```python
from build123d import *

# Parameters (mm, degrees)
SKETCH1_W                = 20
SKETCH1_H                = 15
SWITCHCASE_DEPTH         = 15
SKETCH2_W                = 12.9
SKETCH2_H                = 5.9
SWITCHCAVITY_DEPTH       = 30.154759474
SWITCHM2HOLES_DEPTH      = 28.096171316
SWITCHM2HOLES_DEPTH_BACK = 28.096171316
SKETCH3_R                = 1.05
NUTINSERTS_DEPTH         = 30.154759474
NUTINSERTS_DEPTH_BACK    = 1.75
SKETCH4_W                = 10
SKETCH4_H                = 10
MOUNTTABS_DEPTH          = 2.5
M5SCREWHOLES_REACH       = 36.369
SKETCH6_R                = 2.75
WINGS_DEPTH              = 15
WIRECHANNEL_DEPTH        = 43.884758365
WIRECHANNEL_DEPTH_BACK   = 43.884758365
SKETCH8_W                = 3
SKETCH8_H                = 3
BUMPERCHANNEL_DEPTH      = 46.552167896
BUMPERCHANNEL_DEPTH_BACK = 10.45


with BuildPart() as part:
    # Sketch1 → SwitchCase (new body)
    with BuildSketch(Plane.XY):
        with Locations((10, 7.5)):
            Rectangle(SKETCH1_W, SKETCH1_H)
    extrude(amount=SWITCHCASE_DEPTH)

    # Sketch2 → SwitchCavity (cut, through all)
    with BuildSketch(Plane(origin=(0, 15, 0), x_dir=(1, 0, 0), z_dir=(0, 1, 0))):
        with Locations((10, -7.5)):
            Rectangle(SKETCH2_W, SKETCH2_H)
    extrude(amount=-SWITCHCAVITY_DEPTH, mode=Mode.SUBTRACT)

    # Sketch3 → SwitchM2Holes (cut, two sides: drawn at the far end of the back side and taken through both)
    with BuildSketch(Plane.XY.offset(4.55).offset(-SWITCHM2HOLES_DEPTH_BACK)):
        with Locations((6.7, 8.9)):
            Circle(SKETCH3_R)
        with Locations((13.3, 8.9)):
            Circle(SKETCH3_R)
    extrude(amount=SWITCHM2HOLES_DEPTH + SWITCHM2HOLES_DEPTH_BACK, mode=Mode.SUBTRACT)

    # Sketch5 → NutInserts (cut, two sides: drawn at the far end of the back side and taken through both)
    with BuildSketch(Plane.XY.offset(15).offset(-NUTINSERTS_DEPTH_BACK)):
        Polygon((9.009401077, 8.9), (7.854700538, 10.9), (5.545299462, 10.9), (4.390598923, 8.9), (5.545299462, 6.9), (7.854700538, 6.9), align=None)
        Polygon((15.609401077, 8.9), (14.454700538, 10.9), (12.145299462, 10.9), (10.990598923, 8.9), (12.145299462, 6.9), (14.454700538, 6.9), align=None)
    extrude(amount=NUTINSERTS_DEPTH + NUTINSERTS_DEPTH_BACK, mode=Mode.SUBTRACT)

    # Sketch4 → MountTabs (add)
    with BuildSketch(Plane.XZ):
        with Locations((10, 20)):
            Rectangle(SKETCH4_W, SKETCH4_H)
        with Locations((10, -5)):
            Rectangle(SKETCH4_W, SKETCH4_H)
    extrude(amount=-MOUNTTABS_DEPTH)

    # Sketch6 → M5ScrewHoles (cut, up to next)
    with BuildSketch(Plane(origin=(0, 2.5, 0), x_dir=(1, 0, 0), z_dir=(0, 1, 0)), mode=Mode.PRIVATE) as m5screwholes_sk1:
        with Locations(Location((10, -20, 0), (0, 0, 270))):
            Circle(SKETCH6_R)
    m5screwholes_tool1 = extrude(m5screwholes_sk1.sketch, amount=-M5SCREWHOLES_REACH, mode=Mode.PRIVATE) & part.part
    # Sketch6 → M5ScrewHoles (cut, up to next)
    with BuildSketch(Plane(origin=(0, 2.5, 0), x_dir=(1, 0, 0), z_dir=(0, 1, 0)), mode=Mode.PRIVATE) as m5screwholes_sk2:
        with Locations(Location((10, 5, 0), (0, 0, 270))):
            Circle(SKETCH6_R)
    m5screwholes_tool2 = extrude(m5screwholes_sk2.sketch, amount=-M5SCREWHOLES_REACH, mode=Mode.PRIVATE) & part.part
    add(m5screwholes_tool1.solids().sort_by_distance((10, 2.5, 20))[0], mode=Mode.SUBTRACT)
    add(m5screwholes_tool2.solids().sort_by_distance((10, 2.5, -5))[0], mode=Mode.SUBTRACT)

    # Sketch7 → Wings (add)
    with BuildSketch(Plane.XY.offset(15)):
        Polygon((0, 15), (-15, 15), (-5, 0), (0, 0), align=None)
        Polygon((20, 15), (35, 15), (25, 0), (20, 0), align=None)
    extrude(amount=-WINGS_DEPTH)

    # Sketch8 → WireChannel (cut, two sides: drawn at the far end of the back side and taken through both)
    with BuildSketch(Plane.ZY.offset(-16.45).offset(-WIRECHANNEL_DEPTH_BACK)):
        with Locations((7.5, 1.5)):
            Rectangle(SKETCH8_W, SKETCH8_H)
    extrude(amount=WIRECHANNEL_DEPTH + WIRECHANNEL_DEPTH_BACK, mode=Mode.SUBTRACT)

    # Sketch9 → BumperChannel (cut, two sides: drawn at the far end of the back side and taken through both)
    with BuildSketch(Plane.XY.offset(15).offset(-BUMPERCHANNEL_DEPTH_BACK)):
        Polygon((-9.7, 10.8), (0.55, 10.8), (0.55, 13), (-2.65, 13), (-3.377940469, 15), (-5.772059531, 15), (-6.5, 13), (-9.7, 13), align=None)
        Polygon((26.5, 13), (29.7, 13), (29.7, 10.8), (19.45, 10.8), (19.45, 13), (22.65, 13), (23.377940469, 15), (25.772059531, 15), align=None)
    extrude(amount=BUMPERCHANNEL_DEPTH + BUMPERCHANNEL_DEPTH_BACK, mode=Mode.SUBTRACT)


solid = part.part
```
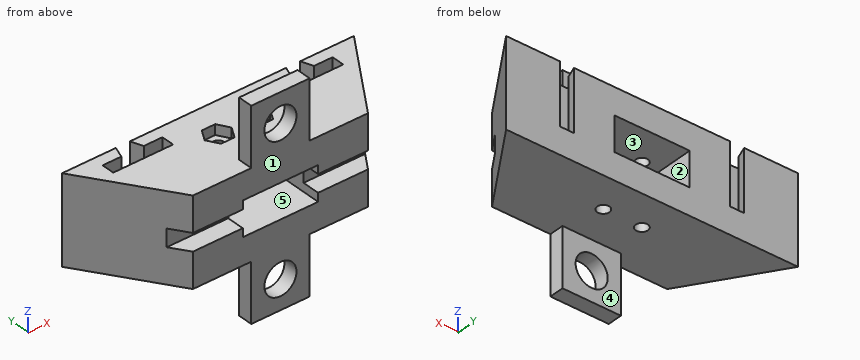
Source: CAD feature listing. Evaluate the final solid. Frame: model axes, mm. Face numbers are marked on the shaded views. A direction names the side the tool comes from. Round coordinates to 2 decimals unless told otherwise and drop trailing zeros. Loops run counter-clockwise (first coordinate to the right, second up) from the corner with the lowest first, then second, coordinate; pieces in that order, holes last. Notation, with made-up numbers: M 84,79 L 90,79 A11 cw 90,93 Z; hole C 8.25,62.25 d9. An arc over 180 degrees is marked long. Use a Markdown table: item, result. Add a question column.
1. Cut plane A-A, the plane z = -5. Output: boundary loops of the cut face in (x, y), and give its area (4 significant figures).
2. Contact query for flat-ended pins moving along their axis: pin 1 (6 mm diameter, centred on y = 6.5, z = -0.5, fed in from -X); pin 2 (1.1 mm diameter, centred on y = 12, z = 10, fed in from -X); pin 3 (2 mm diameter, centred on y = 1.5, z = 22, fed in from -X); pin 4 (1 mm diameter, centred on x = 11, z = -6.5, fed in from +Y). Output: stop coordinate, or through.
3. Set-up query: the marked faces 1 and 2. Return all of +Z, -Z, +X, -X, +Y, -Y with unobstructed straight access to the full face (end or side cutting, diameter ignored); none if empty.
4. Cut plane D-D, the plane z = 3.5. Output: boundary loops of the cut face in (x, y), and give its area (3 significant figures).
5. Cut plane C-C, the plane x = 10. Output: boundary loops of the cut face in (y, z), and give its area (3 significant figures).
6. Cut plane B-B, the plane y = 3.75. Output: boundary loops of the cut face in (x, z), and give its area (3 significant figures).
7. Pull-direction query (Z, two-part tool) for the marked faces 3, 4 and 5; classes: +Z half, -Z half, draft (parallel to the pull), parting line (faces both ways), or undercut.
8. Ray query, line 1 along Y through (x, z) = (13.3, 2.1); line 2 along X through (y, z) = (8.9, 12.5); line 3 along Z through (x, y) = (6, 12.5). Return the intervals inside material, ascending. Write a range as [from, to].
Solution:
| question | item | result |
|---|---|---|
| 1 | outline | M 5,0 L 7.25,0 L 7.25,2.5 L 5,2.5 Z; M 12.75,0 L 15,0 L 15,2.5 L 12.75,2.5 Z |
| 1 | area | 11.25 mm2 |
| 2 | pin 1 | stops at x = -11.31 |
| 2 | pin 2 | stops at x = -13.37 |
| 2 | pin 3 | stops at x = 5 |
| 2 | pin 4 | passes through |
| 3 | face 1 | +Z, -Z, +X, -X, -Y |
| 3 | face 2 | +Y, -Y |
| 4 | outline | M -15,15 L -5,0 L 25,0 L 35,15 Z; hole C 6.7,8.9 d2.1; hole C 13.3,8.9 d2.1 |
| 4 | area | 593 mm2 |
| 5 | outline | M 0,-10 L 2.5,-10 L 2.5,-7.75 L 0,-7.75 Z; M 0,-2.25 L 2.5,-2.25 L 2.5,0 L 15,0 L 15,4.55 L 0,4.55 Z; M 0,10.45 L 15,10.45 L 15,15 L 2.5,15 L 2.5,17.25 L 0,17.25 Z; M 0,22.75 L 2.5,22.75 L 2.5,25 L 0,25 Z |
| 5 | area | 159 mm2 |
| 6 | outline | M -7.5,0 L 27.5,0 L 27.5,15 L -7.5,15 Z; hole M 3.55,4.55 L 16.45,4.55 L 16.45,10.45 L 3.55,10.45 Z |
| 6 | area | 449 mm2 |
| 7 | face 3 | undercut |
| 7 | face 4 | draft |
| 7 | face 5 | undercut |
| 8 | line 1 | y = [0, 7.85], [9.95, 15] |
| 8 | line 2 | x = [-10.93, 5.65], [7.75, 12.25], [14.35, 30.93] |
| 8 | line 3 | z = [0, 4.55], [10.45, 15] |
